Read the model definition and answer for the solid it produces. Units are mm, in the model's axes. A direction names the side the tool comes from. Give positions to 0.01 mm unless a question says otherwise; leave off trailing zeros. Write each loop counter-clockwise with the first axis right and the second up, starting at its lowest first coordinate (ties: lowest second). Pieces come first, ordered by that corner, then holes. Notation, with made-up numbers: (-33.75, -7) -> (12.25, -7) arc R10 ccw to (12.25, 10) -> close; hole circle Ø1 at (-22.5, 15.25). An arc over 180 degrees is marked (long way). Use a Markdown table: item, result.
Autodesk Inventor part; units mm, degrees
ref_plane "YZ Plane" through (0, 0, 0) normal (1, 0, 0) x (0, 1, 0)
ref_plane "XZ Plane" through (0, 0, 0) normal (0, 1, 0) x (-1, 0, 0)
ref_plane "XY Plane" through (0, 0, 0) normal (0, 0, 1) x (1, 0, 0)
sketch "Эскиз1" plane through (0, 0, 0) normal (1, 0, 0) x (0, 1, 0)
  circle A0 centre (0, 0) radius 5.5
  circle A1 centre (0, 0) radius 9
  dimension "d0" = 11
  dimension "d1" = 18
extrude "Выдавливание1" add sketch "Эскиз1" along normal mid plane 2.5
sketch "Эскиз2" plane through (0, 0, 0) normal (1, 0, 0) x (0, 1, 0)
  circle A0 centre (0, 0) radius 9
  circle A1 centre (0, 0) radius 15
  dimension "d4" = 30
extrude "Выдавливание2" add sketch "Эскиз2" along normal mid plane 4.25
properties part number "wheel"
Item 1: Straight lines are drawn through the part: line 1 along Z through (x, y) = (-1.65, 0); line 2 along Z through (x, y) = (0.35, 2.25); line 3 along Y through (x, z) = (1.55, -1.75). For each, find the intervals that lie inside material, in ascending order. Write a range as [from, to].
Return value:
| item | result |
|---|---|
| line 1 | [-15, -9], [9, 15] |
| line 2 | [-14.83, -5.02], [5.02, 14.83] |
| line 3 | [-14.9, -8.83], [8.83, 14.9] |
Item 2: A cutting plane is placed at D-D (y = -8.25). Give the vertices of the cut face in (x, z) (3 decimals), then the cut area to 3 significant figures.
Return value:
| item | result |
|---|---|
| outline | (-2.125, -12.527) -> (2.125, -12.527) -> (2.125, -3.597) -> (1.25, -3.597) -> (1.25, 3.597) -> (2.125, 3.597) -> (2.125, 12.527) -> (-2.125, 12.527) -> (-2.125, 3.597) -> (-1.25, 3.597) -> (-1.25, -3.597) -> (-2.125, -3.597) -> close |
| area | 93.9 mm^2 |
Item 3: A tool of negligible diameter and unlimited length cuts with its end or side. For faces 4 (the face through (1.681, -1.172, -8.923)), 5 (the face through (-0.02, -1.19, 5.37)), 6 (the face through (-1.25, -4, -4)), from which of +Z, -Z, +X, -X, +Y, -Y can it reach the whole face along a straight path? Write none if from no direction.
Return value:
| item | result |
|---|---|
| face 4 | +X |
| face 5 | +X, -X |
| face 6 | -X |
Item 4: A cutting plane is placed at A-A (z = 0). Give the vertices of the cut face in (x, y) (3 decimals).
Return value:
| item | result |
|---|---|
| outline | (-2.125, -15) -> (2.125, -15) -> (2.125, -9) -> (1.25, -9) -> (1.25, -5.5) -> (-1.25, -5.5) -> (-1.25, -9) -> (-2.125, -9) -> close; (-2.125, 9) -> (-1.25, 9) -> (-1.25, 5.5) -> (1.25, 5.5) -> (1.25, 9) -> (2.125, 9) -> (2.125, 15) -> (-2.125, 15) -> close |
Item 5: A cutting plane is placed at C-C (x = 0). Give the vertices of the cut face in (y, z), then the cut area to 3 significant figures.
Return value:
| item | result |
|---|---|
| outline | circle Ø30 at (0, 0); hole circle Ø11 at (0, 0) |
| area | 612 mm^2 |
Item 6: For a pull along Z with two mould halves and no side action, classify faces 1 (the face through (-1.681, -1.172, 8.923)), 2 (the face through (2.125, 6.5, -6.5)), 3 (the face through (0.03, -14.985, 0.66)) as +Z half, -Z half, draft (parallel to the pull), parting line (faces both ways), or undercut.
Return value:
| item | result |
|---|---|
| face 1 | undercut |
| face 2 | draft |
| face 3 | parting line |
Item 7: Each of these flat-tipped pins is pushed along its axis until it touches: P1, Ø14.5, axis at y = 0, z = 0, coming from the -X side; P2, Ø1, axis at x = -1, y = -2, coming from the +Z side; P3, Ø5.5, axis at y = -3.5, z = 3.5, coming from the +X side. Where does it stop, or does it pass through?
Return value:
| item | result |
|---|---|
| P1 | x = -1.25 |
| P2 | z = 14.92 |
| P3 | x = 1.25 |
